Autodesk Inventor part; units mm, degrees
ref_plane "Start Plane" through (0, 0, -4.4541) normal (0, 0, 1) x (1, 0, 0)
ref_plane "End Plane" through (0, 0, 219.0092) normal (0, 0, 1) x (1, 0, 0)
ref_plane "Work Plane4" through (-9.359, -5.1201, -11.1594) normal (0.6341, 0.3469, -0.691) x (-0.3015, -0.712, -0.6341)
ref_plane "Start Plane" through (0, 0, -4.4541) normal (0, 0, 1) x (1, 0, 0)
ref_plane "End Plane" through (0, 0, 219.0092) normal (0, 0, 1) x (1, 0, 0)
sketch "Sketch" plane through (0, 0, 0) normal (0, 0, 1) x (1, 0, 0)
  circle A0 centre (0, 0) radius 6.9342
  circle A1 centre (0, 0) radius 10.668
  dimension "d0" = 21.336
  dimension "d1" = 3.7338
extrude "Body" add sketch "Sketch" along normal up to surface (223.4633 mm away) from surface at -4.4541
sketch "Sketch3" plane through (0, 0, 0) normal (0, 0, 1) x (1, 0, 0)
  line L0 (0, 0) -> (10, 0)
ref_plane "Work Plane3" through (0, 0, 0) normal (0, -1, 0) x (1, 0, 0)
sketch "Sketch4" plane through (0, 0, 0) normal (0, -1, 0) x (1, 0, 0)
  line L0 (-2, -4.4541) -> (12, -4.4541)
  line L1 (-2, 219.0092) -> (12, 219.0092)
  dimension "d7" = 223.4633
ref_plane "Work Plane4" through (-9.359, -5.1201, -11.1594) normal (0.6341, 0.3469, -0.691) x (-0.3015, -0.712, -0.6341)
split "Split1" plane through (-9.359, -5.1201, -11.1594) removes the side toward (0.6341, 0.3469, -0.691)
ref_plane "Work Plane5" through (5.0201, -9.413, -4.8357) normal (-0.1943, 0.3643, -0.9108) x (0.5769, 0.7934, 0.1943)
split "Split2" plane through (5.0201, -9.413, -4.8357) removes the side toward (-0.1943, 0.3643, -0.9108)
ref_plane "Work Plane6" through (8.586, -6.3314, -10.5353) normal (-0.5655, 0.417, -0.7115) x (-0.1087, 0.8175, 0.5655)
split "Split3" plane through (8.586, -6.3314, -10.5353) removes the side toward (-0.5655, 0.417, -0.7115)
ref_plane "Work Plane7" through (-9.359, -5.12, 221.8641) normal (0.6062, 0.3316, 0.7228) x (0.7867, -0.1167, -0.6062)
split "Split4" plane through (-9.359, -5.12, 221.8641) removes the side toward (0.6062, 0.3316, 0.7228)
ref_plane "Work Plane8" through (8.586, -6.3314, 234.1893) normal (-0.7274, 0.5364, 0.4281) x (0.6295, 0.2732, 0.7274)
split "Split5" plane through (8.586, -6.3314, 234.1893) removes the side toward (-0.7274, 0.5364, 0.4281)
ref_plane "Work Plane9" through (6.001, -8.8201, 225.8384) normal (-0.4494, 0.6606, 0.6014) x (0.8739, 0.1854, 0.4494)
split "Split6" plane through (6.001, -8.8201, 225.8384) removes the side toward (-0.4494, 0.6606, 0.6014)
equation "\"d0\" = G_H"
equation "\"d1\" = G_T"
equation "\"d2\" = G_L"
equation "\"G_H\" = 21.336"
equation "\"G_T\" = 3.7338"
equation "\"G_L\" = 223.46333"
equation "\"G_OFFSET_START\" = 4.45413"
equation "\"G_OFFSET_END\" = 7.34335"
equation "\"d4\" = -G_OFFSET_START"
equation "\"d5\" = G_OFFSET_END + B_L"
equation "\"B_L\" = 211.66585"
properties part number "ANSI - 1/2 x 0.147 - 8.798" material "Steel, Mild"
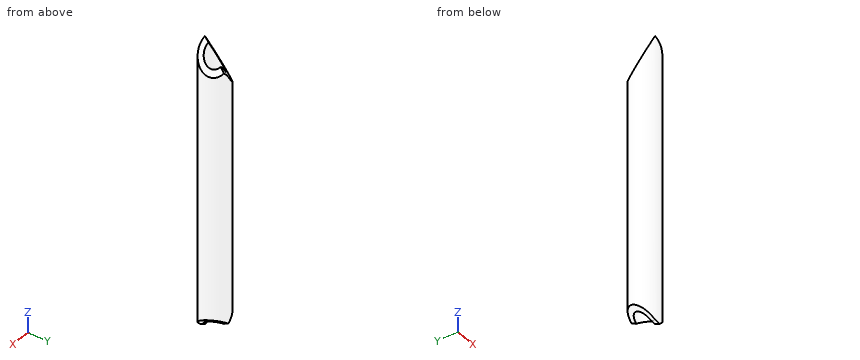
Design review of the part built by this model. Coordinates are the model's own, in mm. Coordinates: 2 decimals unless noted, no trailing zeros. Loops run counter-clockwise (first coordinate to the right, second up) from the corner with the lowest first, then second, coordinate; pieces in that order, holes last. Notation, with made-up numbers: (46.25, -32.75) -> (82.25, -32.75) arc R26 ccw to (82.25, -4.75) -> close; hole circle Ø7 at (13.25, -28). An arc over 180 degrees is marked (long way). Answer as a JSON object with one key per item and string values.
Q1. To check wall thickness, follow L1, parallel to X at y = 0, z = 134; L2, parallel to X at y = -6, z = 89. State the ranges of each line that lie inside material, in increasing order.
Answer block:
{"L1": "x = -10.67 to -6.93, 6.93 to 10.67", "L2": "x = -8.82 to -3.48, 3.48 to 8.82"}
Q2. Take a section at A-A on y = -2.5. Give the boundary of the cut face in (x, z), plus the area to 3 significant figures.
Answer block:
{"outline": "(-10.37, 6.78) -> (-6.47, 3.68) -> (-6.47, 203.81) -> (-10.37, 197.18) -> close; (6.47, 4.68) -> (10.37, 8.26) -> (10.37, 204.11) -> (6.47, 207.39) -> close", "area": "1,540 mm^2"}
Q3. Clearance check with flat-ended pins moving along their axes: pin 1 Ø8 at (y, z) = (-4, 26.5) entering from +X; pin 2 Ø4 at (y, z) = (6.5, 70.5) entering from +X; pin 3 Ø2 at (x, y) = (-2.5, -6) entering from +Z; pin 4 Ø6 at (x, z) = (6, 147.5) entering from -Y. State where each tip first meets the part, or that it passes through.
Answer block:
{"pin 1": "stops at x = 10.67", "pin 2": "stops at x = 9.67", "pin 3": "stops at z = 216.68", "pin 4": "stops at y = -10.24"}
